The model under review builds one solid part; all positions refer to its coordinate system, in mm. A direction names the side the tool comes from. Give positions to 0.01 mm unless a question says otherwise; leave off trailing zeros. Order: outer loops, then holes, each group sorted by start corner. A loop starts at its lowest first (then second) coordinate and runs counter-clockwise, first axis right, second up. Notation, with made-up numbers: (77.25, 30.5) - (130.25, 30.5) arc R35 cw to (130.25, 66.5) - close; hole circle Ø6 at (22.25, 42). An arc over 180 degrees is marked (long way). Put each result on its own line as item: value.
```python
from build123d import *

# Parameters (mm, degrees)
F1_DEPTH = 63.5
F0_W     = 23.213864
F0_H     = 19.05
F2_DEPTH = 25.4
F3_DEPTH = 7.9375
F0_W_2   = 25.4
F0_H_2   = 28.575
F5_R     = 6.35


with BuildPart() as f1:
    # F0 (on Front) → F1 (new body, symmetric)
    with BuildSketch(Plane.XZ):
        Polygon((-41.275, -9.525), (41.275, -9.525), (41.275, 9.525), (22.225, 9.525), (-41.275, 9.525), align=None)
    extrude(amount=F1_DEPTH, both=True)

    # F0 (on Front) → F2 (join, symmetric)
    with BuildSketch(Plane.XZ):
        with BuildLine():
            Line((22.225, 9.525), (41.275, 9.525))
            Line((41.275, 9.525), (41.275, 26.632201))
            ThreePointArc((41.275, 26.632201), (45.791052, 38.09465), (57.145734, 42.8752))
            Line((57.145734, 42.8752), (60.325, 42.8752))
            Line((60.325, 42.8752), (60.325, 61.9252))
            Line((60.325, 61.9252), (57.145734, 61.9252))
            add(Edge.make_bspline(
                [(54.854475, 61.84996), (55.629553, 61.887449), (56.393583, 61.912637), (57.145734, 61.9252)],
                knots=[109.150564, 109.150564, 109.150564, 109.150564, 111.500771, 111.500771, 111.500771, 111.500771], degree=3))
            ThreePointArc((54.854475, 61.84996), (31.467038, 50.672129), (22.225, 26.454349))
            Line((22.225, 26.454349), (22.225, 9.525))
        make_face()
        with Locations((71.931932, 52.4002)):
            Rectangle(F0_W, F0_H)
    extrude(amount=F2_DEPTH, both=True)

    # F0 (on Front) → F3 (join, symmetric)
    with BuildSketch(Plane.XZ):
        with BuildLine():
            add(Edge.make_bspline(
                [(-41.275, 9.525), (-40.968024, 31.835338), (18.857574, 60.108855), (54.854475, 61.84996)],
                knots=[0, 0, 0, 0, 109.150564, 109.150564, 109.150564, 109.150564], degree=3))
            Line((-41.275, 9.525), (22.225, 9.525))
            Line((22.225, 9.525), (22.225, 26.454349))
            ThreePointArc((22.225, 26.454349), (31.467038, 50.672129), (54.854475, 61.84996))
        make_face()
    extrude(amount=F3_DEPTH, both=True)

    # F0 (on Front) → F4 (revolve)
    with BuildSketch(Plane.XZ):
        with Locations((98.425, 52.3875)):
            Rectangle(F0_W_2, F0_H_2)
    revolve(axis=Axis((85.725, 0, 52.3875), (0, 0, 1)))

    # F5
    f5_edges = [f1.edges().sort_by_distance(p)[0] for p in [
        (-41.275, -63.5, 0),
        (41.275, -63.5, 0),
        (41.275, 63.5, 0),
        (-41.275, 63.5, 0),
    ]]
    fillet(f5_edges, radius=F5_R)


solid = f1.part
```
(1) For faces 4 (the flat face through (41.275, -1, 4)), 5 (the flat face through (22.225, -17, 18)), 6 (the flat face through (46, -25.4, 42)), 7 (the flat face through (60, -2, 61.925)), list the 3-axis set-ups (+Z, -Z, +X, -X, +Y, -Y) from which the entire face can be reached by the end or side of a thin tool; tool diameter is ignored.
The answers:
face 4: -Z, +X, +Y, -Y
face 5: +Z, -X, -Y
face 6: +Z, +X, -X, -Y
face 7: +Z, -X
(2) Take a section at D-D, the plane x = 79. Write out the cut boundary in (y, z) (3 decimals).
The answers:
outline: (-25.4, 42.875) - (-24.494, 42.875) - (-24.494, 38.1) - (24.494, 38.1) - (24.494, 42.875) - (25.4, 42.875) - (25.4, 61.925) - (24.494, 61.925) - (24.494, 66.675) - (-24.494, 66.675) - (-24.494, 61.925) - (-25.4, 61.925) - close
(3) Wall thickness on L1, parallel to Z at x = -6, y = 53.5 (3 decimals); L2, parallel to X at y = -49, z = -5 (3 decimals); L3, parallel to Z at x = 57, y = 15: over which ranges is each line inside the solid? List them lowest first.
The answers:
L1: -9.525 to 9.525
L2: -41.275 to 41.275
L3: 42.87 to 61.92
(4) Take a section at B-B, the plane y = 29. Write out the cut boundary in (x, z) (3 decimals).
The answers:
outline: (-41.275, -9.525) - (41.275, -9.525) - (41.275, 9.525) - (-41.275, 9.525) - close
(5) Take a section at A-A, the plane z = 1. Write out the cut boundary in (x, y) (3 decimals).
The answers:
outline: (-41.275, -57.15) arc R6.35 ccw to (-34.925, -63.5) - (34.925, -63.5) arc R6.35 ccw to (41.275, -57.15) - (41.275, 57.15) arc R6.35 ccw to (34.925, 63.5) - (-34.925, 63.5) arc R6.35 ccw to (-41.275, 57.15) - close
(6) Take a section at C-C, the plane x = 62.5. Write out the cut boundary in (y, z) (3 decimals).
The answers:
outline: (-25.4, 42.875) - (-10.284, 42.875) - (-10.284, 38.1) - (10.284, 38.1) - (10.284, 42.875) - (25.4, 42.875) - (25.4, 61.925) - (10.284, 61.925) - (10.284, 66.675) - (-10.284, 66.675) - (-10.284, 61.925) - (-25.4, 61.925) - close
(7) Clearance check with flat-ended pins moving along their axes: pin 1 Ø3 at (x, y) = (70, -24) entering from +Z; pin 2 Ø15.5 at (x, z) = (19, 23.5) entering from -Y; pin 3 Ø13.5 at (y, z) = (20, 19.5) entering from -X (3 decimals). State where each tip first meets the part, or that it passes through.
The answers:
pin 1: z = 61.93
pin 2: y = -25.4
pin 3: x = 22.225
(8) The part is to be moulded in two halves that separate along X. For faces 1 (the flat face through (-3, -7.938, 30)), 2 (the flat face through (60, 2, 42.875)), 3 (the cylindrical face through (39.464, 61.59, 0.133)), say which applies: pulls with the +X half, pulls with the -X half, needs draft (parallel to the pull), parting line crosses it, or undercut.
The answers:
face 1: needs draft
face 2: undercut
face 3: pulls with the +X half
